Source: CAD feature listing. Evaluate the final solid. Frame: model axes, mm. Coordinates: 2 decimals unless noted, no trailing zeros. Order: outer loops, then holes, each group sorted by start corner. A loop starts at its lowest first (then second) coordinate and runs counter-clockwise, first axis right, second up.
Item 1: Section A-A on z = 6.25. State how many separate pieces and enclosed holes the cut face has, then the cut area to 3 significant figures.
Item 2: Ray query, line 1 (Y direction, x = 17.75, z = 5.25); line 2 (Y direction, x = 8.5, z = 5.5). Return the intervals inside material, ascending.
Item 3: Section B-B on x = 16. Return the cut outline in (y, z).
Item 4: Contact query for a flat-ended pin moving along its axis: P1, Ø0.5, axis at x = 11, y = 2, coming from the +Z side. Output: stop coordinate, or through.
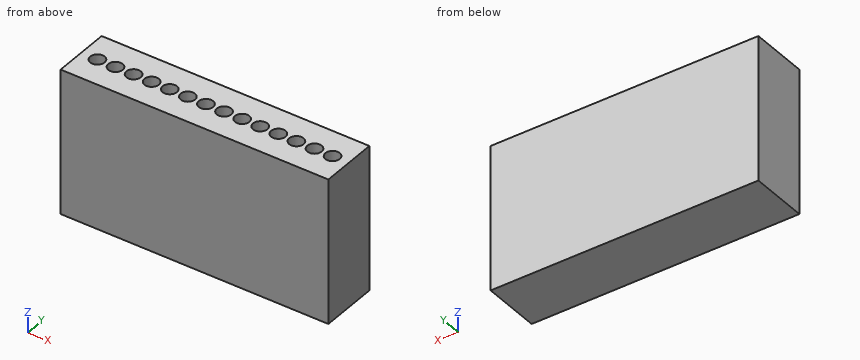
from build123d import *

# Parameters (mm, degrees)
SKETCH2_W           = 18.5
SKETCH2_H           = 4
BOSS_EXTRUDE1_DEPTH = 10
SKETCH3_R           = 0.5
CUT_EXTRUDE1_DEPTH  = 5


with BuildPart() as part:
    # Sketch2 → Boss-Extrude1 (new body)
    with BuildSketch(Plane.XY):
        with Locations((9.25, 2)):
            Rectangle(SKETCH2_W, SKETCH2_H)
    extrude(amount=BOSS_EXTRUDE1_DEPTH)

    # Sketch3 → Cut-Extrude1 (cut)
    with BuildSketch(Plane.XY.offset(10)):
        with Locations((1.125, 2)):
            Circle(SKETCH3_R)
        with Locations((2.375, 2)):
            Circle(SKETCH3_R)
        with Locations((3.625, 2)):
            Circle(SKETCH3_R)
        with Locations((4.875, 2)):
            Circle(SKETCH3_R)
        with Locations((6.125, 2)):
            Circle(SKETCH3_R)
        with Locations((7.375, 2)):
            Circle(SKETCH3_R)
        with Locations((8.625, 2)):
            Circle(SKETCH3_R)
        with Locations((9.875, 2)):
            Circle(SKETCH3_R)
        with Locations((11.125, 2)):
            Circle(SKETCH3_R)
        with Locations((12.375, 2)):
            Circle(SKETCH3_R)
        with Locations((13.625, 2)):
            Circle(SKETCH3_R)
        with Locations((14.875, 2)):
            Circle(SKETCH3_R)
        with Locations((16.125, 2)):
            Circle(SKETCH3_R)
        with Locations((17.375, 2)):
            Circle(SKETCH3_R)
    extrude(amount=-CUT_EXTRUDE1_DEPTH, mode=Mode.SUBTRACT)


solid = part.part
Answer list:
1. separate pieces: 1
1. enclosed holes: 14
1. area: 63.0 mm2
2. line 1: y = 0 to 1.67, 2.33 to 4
2. line 2: y = 0 to 1.52, 2.48 to 4
3. outline: (0, 0) - (4, 0) - (4, 10) - (2.48, 10) - (2.48, 5) - (1.52, 5) - (1.52, 10) - (0, 10) - close
4. P1: stops at z = 5
